```python
from build123d import *

# Parameters (mm, degrees)
DODANIE_WYCI_GNI_CIE1_DEPTH      = 2.6
SZKIC4_R                         = 2
WYTNIJ_WYCI_GNI_CIE1_DEPTH       = 2.6
SZKIC5_W                         = 49.1
SZKIC5_H                         = 14.2
DODANIE_WYCI_GNI_CIE3_DEPTH      = 5.3
DODANIE_WYCI_GNI_CIE4_DEPTH      = 49.1
SZKIC10_R                        = 1
DODANIE_WYCI_GNI_CIE5_DEPTH      = 11.7
DODANIE_WYCI_GNI_CIE5_DEPTH_BACK = 60.8


with BuildPart() as part:
    # Szkic1 → Dodanie-wyciągnięcie1 (new body)
    with BuildSketch(Plane(origin=(0, 0, 0), x_dir=(1, 0, 0), z_dir=(0, 1, 0))):
        Polygon((0, 0), (0, 21.95), (39.7, 21.95), (39.7, 29.7), (49.1, 29.7), (49.1, 7.75), (9.4, 7.75), (9.4, 0), align=None)
    extrude(amount=DODANIE_WYCI_GNI_CIE1_DEPTH)

    # Szkic4 → Wytnij-wyciągnięcie1 (cut)
    with BuildSketch(Plane.XZ):
        with Locations((4.7, -4.15)):
            Circle(SZKIC4_R)
        with Locations((44.4, -25.55)):
            Circle(SZKIC4_R)
    extrude(amount=-WYTNIJ_WYCI_GNI_CIE1_DEPTH, mode=Mode.SUBTRACT)

    # Szkic5 → Dodanie-wyciągnięcie3 (add)
    with BuildSketch(Plane(origin=(0, 2.6, 0), x_dir=(1, 0, 0), z_dir=(0, 1, 0))):
        with Locations((24.55, 14.85)):
            Rectangle(SZKIC5_W, SZKIC5_H)
    extrude(amount=DODANIE_WYCI_GNI_CIE3_DEPTH)

    # Szkic7 → Dodanie-wyciągnięcie4 (add)
    with BuildSketch(Plane(origin=(0, 0, 0), x_dir=(0, 0, -1), z_dir=(1, 0, 0))):
        with BuildLine():
            Line((13.176679947, 14.8), (16.523320053, 14.8))
            ThreePointArc((16.523320053, 14.8), (14.85, 0.8), (13.176679947, 14.8))
        make_face()
    extrude(amount=DODANIE_WYCI_GNI_CIE4_DEPTH)

    # Szkic10 → Dodanie-wyciągnięcie5 (add, two sides)
    with BuildSketch(Plane.ZY) as dodanie_wyci_gni_cie5_sk:
        with Locations((-14.85, 7.9)):
            Circle(SZKIC10_R)
    extrude(amount=DODANIE_WYCI_GNI_CIE5_DEPTH)
    extrude(dodanie_wyci_gni_cie5_sk.sketch, amount=-DODANIE_WYCI_GNI_CIE5_DEPTH_BACK)


solid = part.part
```
Could you check a few things on this model? Use its own coordinates, in mm. A direction names the side the tool comes from. Coordinates: 2 decimals unless noted, no trailing zeros. Write each loop counter-clockwise with the first axis right and the second up, starting at its lowest first coordinate (ties: lowest second). Pieces come first, ordered by that corner, then holes. Notation, with made-up numbers: M 23,83.5 L 27,83.5 A17 ccw 27,100.5 Z; hole C -5.5,-18 d2. An arc over 180 degrees is marked long. Answer as CSV lines item,"result". Start each with the question number.
1) We'd pull the mould along X, two halves only. Please class faces 4 (the flat face through (-11.7, 8, -15)), 5 (the cylindrical face through (42.4, 1.3, -25.5)), 6 (the cylindrical face through (-5.77, 7.29, -15.64)): +X half, -X half, draft (parallel to the pull), parting line (faces both ways), or undercut.
2) I want a section at B-B, the plane x = 4.7. Please give me the cut outline in (y, z), and give its area (3 significant figures).
3) I want a section at C-C, the plane x = 48. Please give me the cut outline in (y, z).
4) For P1, Ø2.5, axis at x = 3, z = -5, coming from the +Y side; P2, Ø3, axis at y = 5.5, z = -18.5, coming from the +X side; P3, Ø1, axis at y = 9, z = -18.5, coming from the -X side; P4, Ø2.5, axis at x = 4.7, z = -4.15, coming from the +Y side, each with a flat end and sliding along its axis, tell me the tip position at first contact or that it passes through.
5) For faces 1 (the flat face through (44, 2.6, -28)), 2 (the cylindrical face through (54.87, 7.29, -15.64)), 3 (the flat face through (39.7, 1, -26)), which set-ups out of +Z, -Z, +X, -X, +Y, -Y let a thin tool reach every point of the face, with its end or its side?
6) I want a section at A-A, the plane z = -4.15. Please give me the cut outline in (x, y).
7) Please list where these lines run through material, in increasing order: line 1 (Z direction, x = 4.7, y = 1.6); line 2 (Z direction, x = 44.4, y = 2); line 3 (Z direction, x = 8, y = 2). Write a range as from..to.
8) I want a section at D-D, the plane z = -14.85. Please give me the cut outline in (x, y).
Data:
1,face 4,"-X half"
1,face 5,"undercut"
1,face 6,"draft"
2,outline,"M 0,-21.95 L 7.9,-21.95 A7.1 ccw 14.8,-16.52 L 14.8,-13.18 A7.1 ccw 7.9,-7.75 L 2.6,-7.75 L 2.6,-6.15 L 0,-6.15 Z; M 0,-2.15 L 2.6,-2.15 L 2.6,0 L 0,0 Z"
2,area,"201 mm^2"
3,outline,"M 0,-29.7 L 2.6,-29.7 L 2.6,-21.95 L 7.9,-21.95 A7.1 ccw 14.8,-16.52 L 14.8,-13.18 A7.1 ccw 7.9,-7.75 L 0,-7.75 Z"
4,P1,"stops at y = 2.6"
4,P2,"stops at x = 49.1"
4,P3,"stops at x = 0"
4,P4,"passes through"
5,face 1,"-Z, +X, -X, +Y"
5,face 2,"+X"
5,face 3,"-Z, -X, +Y, -Y"
6,outline,"M 0,0 L 2.7,0 L 2.7,2.6 L 0,2.6 Z; M 6.7,0 L 9.4,0 L 9.4,2.6 L 6.7,2.6 Z"
7,line 1,"z = -21.95..-6.15, -2.15..0"
7,line 2,"z = -29.7..-27.55, -23.55..-7.75"
7,line 3,"z = -21.95..0"
8,outline,"M -11.7,6.9 L 0,6.9 L 0,0 L 49.1,0 L 49.1,6.9 L 60.8,6.9 L 60.8,8.9 L 49.1,8.9 L 49.1,14.8 L 0,14.8 L 0,8.9 L -11.7,8.9 Z"
